Source: CAD feature listing. Evaluate the final solid. Frame: model axes, mm. Face numbers are marked on the shaded views. A direction names the side the tool comes from. Give positions to 0.01 mm unless a question says otherwise; leave off trailing zeros. Write each loop counter-clockwise with the first axis right and the second up, starting at its lowest first coordinate (ties: lowest second). Pieces come first, ordered by that corner, then holes. Notation, with made-up numbers: (52, 15) -> (63, 15) arc R14 cw to (63, 34) -> close; hole circle Ø6 at (-14.5, 3). An arc over 180 degrees is marked (long way). Use a Markdown table: item, result. Add a question column.
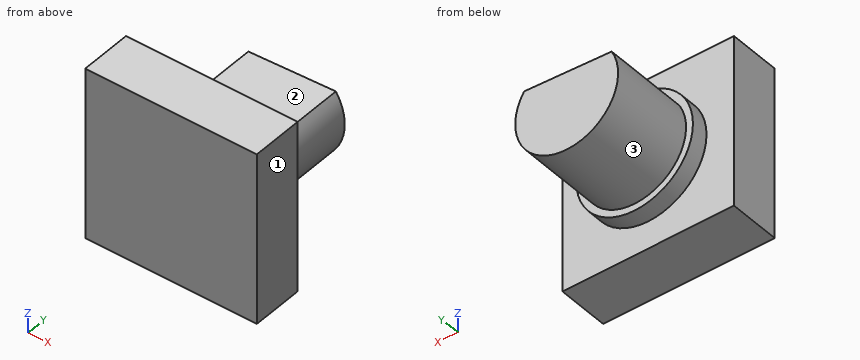
```python
from build123d import *

# Parameters (mm, degrees)
SKETCH_1_W      = 10
SKETCH_1_H      = 10
EXTRUDE_1_DEPTH = 3
SKETCH_2_R      = 3.4
EXTRUDE_2_DEPTH = 1
EXTRUDE_3_DEPTH = 5


with BuildPart() as part:
    # 草图1 → 凸台-拉伸1 (new body)
    with BuildSketch(Plane(origin=(0, 0, 0), x_dir=(1, 0, 0), z_dir=(0, 1, 0))):
        with Locations((-0.373134328, -2.350746269)):
            Rectangle(SKETCH_1_W, SKETCH_1_H)
    extrude(amount=EXTRUDE_1_DEPTH)

    # 草图2 → 凸台-拉伸2 (add)
    with BuildSketch(Plane(origin=(0, 3, 0), x_dir=(1, 0, 0), z_dir=(0, 1, 0))):
        with Locations(Location((-0.373134328, -2.350746269, 0), (0, 0, 270))):
            Circle(SKETCH_2_R)
    extrude(amount=EXTRUDE_2_DEPTH)

    # 草图3 → 凸台-拉伸3 (add)
    with BuildSketch(Plane(origin=(0, 4, 0), x_dir=(1, 0, 0), z_dir=(0, 1, 0))):
        with BuildLine():
            Line((-2.997411901, -3.804419967), (2.106902355, -4.038768203))
            ThreePointArc((2.106902355, -4.038768203), (-0.235543876, 0.646096882), (-2.997411901, -3.804419967))
        make_face()
    extrude(amount=EXTRUDE_3_DEPTH)


solid = part.part
```
(1) Access query for the marked faces 1, 2 and 3. Directions: +Z, -Z, +X, -X, +Y, -Y. A direction counts if a zero-diameter tool reaches every point of the face in a straight line with its end or side. Return the directions, or none.
(2) First-contact query: pin 1 Ø1 at (x, y) = (-3, 5.5) entering from -Z (3 decimals); pin 2 Ø4 at (y, z) = (5.5, -0.5) entering from +X. Flat tips, straight axial feed; report the tip coordinate or a pass-through.
(3) Cut plane A-A on x = 1.25. Return the cut outline in (y, z).
(4) Material intervals for L1, parallel to Y at x = -3.75, z = 0.5; L2, parallel to X at y = 5.5, z = 2.5; L3, parallel to X at y = 5, z = 3.5, sorted ascending.
(5) Cut plane C-C on y = 5.75. Return the cut outline in (x, z), then the cut area to 3 significant figures.
(6) Cut plane B-B on z = 3.25. Return the cut outline in (x, y), then the cut area to 3 significant figures.
(7) Cut plane D-D on z = -1.75. Return the cut outline in (x, y), then the cut area to 3 significant figures.
Output:
| question | item | result |
|---|---|---|
| 1 | face 1 | +Z, -Z, +X, +Y, -Y |
| 1 | face 2 | +Z, -X, +Y |
| 1 | face 3 | +Y |
| 2 | pin 1 | z = 0.235 |
| 2 | pin 2 | x = 2.66 |
| 3 | outline | (0, -2.65) -> (3, -2.65) -> (3, -0.64) -> (4, -0.64) -> (4, -0.17) -> (9, -0.17) -> (9, 4) -> (4, 4) -> (4, 5.34) -> (3, 5.34) -> (3, 7.35) -> (0, 7.35) -> close |
| 4 | L1 | 0 to 3 |
| 4 | L2 | -3.37 to 2.62 |
| 4 | L3 | -3.14 to 2.4 |
| 5 | outline | (-3, 3.8) arc R3 ccw (long way) to (2.11, 4.04) -> close |
| 5 | area | 23.1 mm^2 |
| 6 | outline | (-5.37, 0) -> (4.63, 0) -> (4.63, 3) -> (2.91, 3) -> (2.91, 4) -> (2.49, 4) -> (2.49, 9) -> (-3.24, 9) -> (-3.24, 4) -> (-3.65, 4) -> (-3.65, 3) -> (-5.37, 3) -> close |
| 6 | area | 65.2 mm^2 |
| 7 | outline | (-5.37, 0) -> (4.63, 0) -> (4.63, 3) -> (-5.37, 3) -> close |
| 7 | area | 30.0 mm^2 |
